Geometry: final body of the model. Coordinates: model frame, mm. Face numbers are marked on the shaded views. A direction names the side the tool comes from. Coordinates: 2 decimals unless noted, no trailing zeros. Order: outer loops, then holes, each group sorted by start corner. A loop starts at its lowest first (then second) coordinate and runs counter-clockwise, first axis right, second up. Notation, with made-up numbers: (3.5, 18.5) - (11.5, 18.5) arc R21 cw to (11.5, 27.5) - close; hole circle Ø3 at (51, 77). An arc over 180 degrees is marked (long way). Use one line per item in the form item = value. Start each with the question number.
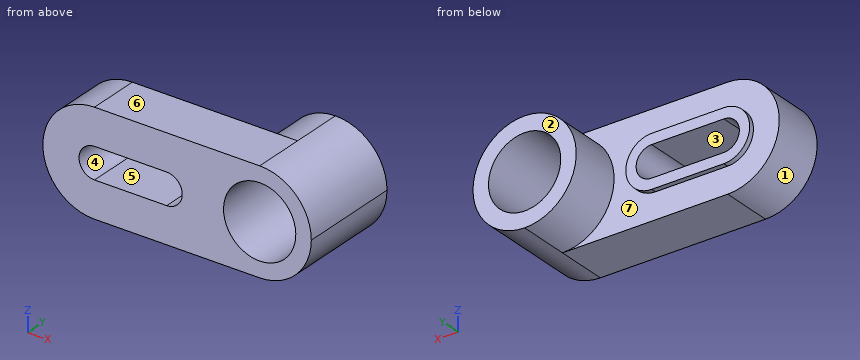
```python
from build123d import *

# Parameters (mm, degrees)
EXTRUDE_1_DEPTH = 10
SKETCH_1_5_R    = 7
EXTRUDE_2_DEPTH = 20
EXTRUDE_3_DEPTH = 11


with BuildPart() as part:
    # Sketch 1 → Extrude 1 (new body)
    with BuildSketch(Plane(origin=(0, 0, 0), x_dir=(1, 0, 0), z_dir=(0, 1, 0))):
        with BuildLine():
            Line((25.09623431, 10), (-6.90376569, 10))
            ThreePointArc((-6.90376569, 10), (-16.90376569, 0), (-6.90376569, -10))
            Line((-6.90376569, -10), (25.09623431, -10))
            ThreePointArc((25.09623431, -10), (15.09623431, 0), (25.09623431, 10))
        make_face()
        with BuildLine():
            ThreePointArc((-6.90376569, -5), (-11.90376569, 0), (-6.90376569, 5))
            Line((-6.90376569, 5), (7.09623431, 5))
            ThreePointArc((7.09623431, 5), (12.09623431, 0), (7.09623431, -5))
            Line((7.09623431, -5), (-6.90376569, -5))
        make_face(mode=Mode.SUBTRACT)
    extrude(amount=EXTRUDE_1_DEPTH)

    # Sketch 1_5 → Extrude 2 (add)
    with BuildSketch(Plane(origin=(0, 0, 0), x_dir=(1, 0, 0), z_dir=(0, 1, 0))):
        with BuildLine():
            ThreePointArc((35.09623431, 0), (32.167302121, 7.071067812), (25.09623431, 10))
            ThreePointArc((25.09623431, 10), (15.09623431, 0), (25.09623431, -10))
            ThreePointArc((25.09623431, -10), (32.167302121, -7.071067812), (35.09623431, 0))
        make_face()
        with Locations(Location((25.09623431, 0, 0), (0, 0, 270))):
            Circle(SKETCH_1_5_R, mode=Mode.SUBTRACT)
    extrude(amount=EXTRUDE_2_DEPTH)

    # Sketch 1_6 → Extrude 3 (add)
    with BuildSketch(Plane(origin=(0, 0, 0), x_dir=(1, 0, 0), z_dir=(0, 1, 0))):
        with BuildLine():
            Line((-6.90376569, 5), (7.09623431, 5))
            ThreePointArc((7.09623431, 5), (12.09623431, 0), (7.09623431, -5))
            Line((7.09623431, -5), (-6.90376569, -5))
            ThreePointArc((-6.90376569, -5), (-11.90376569, 0), (-6.90376569, 5))
        make_face()
        with BuildLine():
            Line((-6.90376569, 3), (7.09623431, 3))
            ThreePointArc((7.09623431, 3), (10.09623431, 0), (7.09623431, -3))
            Line((7.09623431, -3), (-6.90376569, -3))
            ThreePointArc((-6.90376569, -3), (-9.90376569, 0), (-6.90376569, 3))
        make_face(mode=Mode.SUBTRACT)
    extrude(amount=EXTRUDE_3_DEPTH)


solid = part.part
```
(1) Set-up query: the marked faces 5, 6 and 7. Return all of +Z, -Z, +X, -X, +Y, -Y with unobstructed straight access to the full face (end or side cutting, diameter ignored); none if empty.
(2) Draft query along X for the marked faces 1, 2, 3 and 4. Return one class per face: released by +X, released by -X, zero draft, split by the parting line, or undercut.
(3) Cut plane A-A on y = 2.5. Return the cut outline in (x, z).
(4) Cut plane C-C on z = 1.75. Return the cut outline in (x, y).
(5) Material intervals for L1, parallel to Z at x = 2, y = 3.5; L2, parallel to X at y = 3.75, z = -1.5; L3, parallel to X at y = 7.25, z = -2.75, sorted ascending. Write a range as from..to.
(6) Contact query for flat-ended pins moving along their axis: pin 1 Ø0.8 at (x, y) = (-1.5, 10.5) entering from -Z; pin 2 Ø11 at (x, z) = (5, -1) entering from +Y; pin 3 Ø10 at (x, y) = (-4, 17.5) entering from -Z; pin 4 Ø0.5 at (x, y) = (-1.5, 10.5) entering from +Z. Output: stop coordinate, or through.
(7) Cut plane D-D on y = 17.25. Return the cut outline in (x, z), plus the area to 3 significant figures.
(8) Cut plane B-B on x = 8.5. Return the cut outline in (y, z), plus the area to 3 significant figures.
Check sheet entries:
q1.face_5 = +Y, -Y
q1.face_6 = +Z, +X, -X, +Y, -Y
q1.face_7 = +Y
q2.face_1 = released by -X
q2.face_2 = zero draft
q2.face_3 = undercut
q2.face_4 = undercut
q3.outline = (-6.9, -10) - (25.1, -10) arc R10 ccw to (25.1, 10) - (-6.9, 10) arc R10 ccw to start; hole (-6.9, -3) - (7.1, -3) arc R3 ccw to (7.1, 3) - (-6.9, 3) arc R3 ccw to start; hole circle Ø14 at (25.1, 0)
q4.outline = (-16.75, 0) - (-9.34, 0) - (-9.34, 11) - (-11.59, 11) - (-11.59, 10) - (-16.75, 10) - close; (9.53, 0) - (18.32, 0) - (18.32, 20) - (15.25, 20) - (15.25, 10) - (11.78, 10) - (11.78, 11) - (9.53, 11) - close; (31.87, 0) - (34.94, 0) - (34.94, 20) - (31.87, 20) - close
q5.L1 = -10..-3, 3..10
q5.L2 = -16.79..-9.5, 9.69..18.26, 31.93..34.98
q5.L3 = -16.52..-8.1, 8.3..18.66, 31.53..34.71
q6.pin_1 = -5
q6.pin_2 = 11
q6.pin_3 = through
q6.pin_4 = 5
q7.outline = circle Ø20 at (25.1, 0); hole circle Ø14 at (25.1, 0)
q7.area = 160 mm^2
q8.outline = (0, -10) - (10, -10) - (10, -4.8) - (11, -4.8) - (11, -2.65) - (0, -2.65) - close; (0, 2.65) - (11, 2.65) - (11, 4.8) - (10, 4.8) - (10, 10) - (0, 10) - close
q8.area = 151 mm^2
